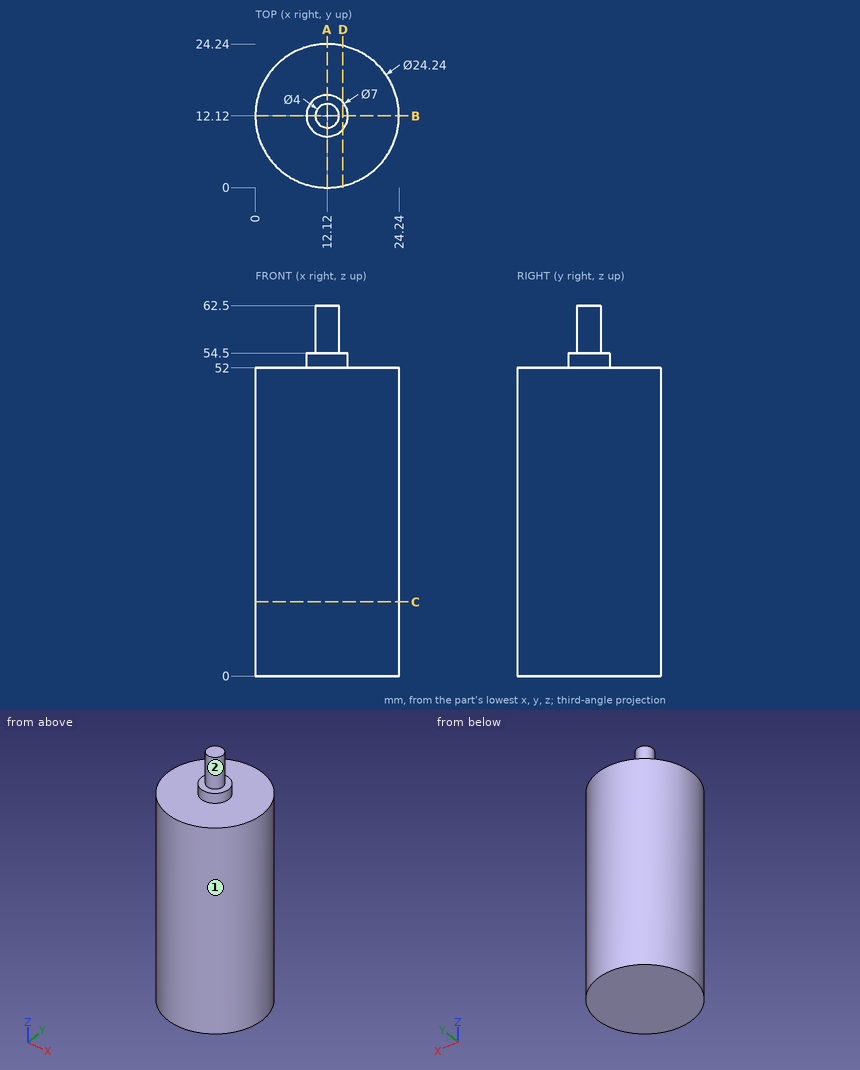
The figure shows three views and two pictorial views of one solid part (mm, origin at its lowest corner). Answer the questions. A direction names the side the tool comes from. Give positions to 0.01 mm unless a question says otherwise; leave off trailing zeros. Loops run counter-clockwise (first coordinate to the right, second up) from the corner with the lowest first, then second, coordinate; pieces in that order, holes last. Notation, with made-up numbers: (55.5, 42) -> (98.5, 42) arc R15 cw to (98.5, 61) -> close; hole circle Ø6 at (-23, 26.25). An arc over 180 degrees is marked (long way). Put each result on its own line as item: value. Start each with the question number.
Item 1: Which of the six approach directions +Z, -Z, +X, -X, +Y, -Y give full straight-line access (tool end or side, diameter ignored) to the marked faces 1 and 2?
Item 2: The part is cut by section A-A (x = 12.12). Give the vertices of the cut face in (y, z).
Item 3: Find the intervals of material crossed by L1, parallel to Z at x = 9.5, y = 11; L2, parallel to X at y = 12.5, z = 13.5; L3, parallel to Z at x = 5.75, y = 20.5, in increasing order. Write a range as [from, to].
Item 4: The part is cut by section C-C (z = 12.5). Give the vertices of the cut face in (x, y).
Item 5: Each of these flat-tipped pins is pushed along its axis until it touches: P1, Ø8, axis at x = 17.5, z = 49.5, coming from the +Y side; P2, Ø1.5, axis at y = 18, z = 9.5, coming from the +X side. Where does it stop, or does it pass through?
Item 6: The part is cut by section D-D (x = 14.75). Give the vertices of the cut face in (y, z), then the cut area to 3 significant figures.
Answers below:
1. face 1: +Z, -Z
1. face 2: +Z
2. outline: (0, 0) -> (24.24, 0) -> (24.24, 52) -> (15.62, 52) -> (15.62, 54.5) -> (14.12, 54.5) -> (14.12, 62.5) -> (10.12, 62.5) -> (10.12, 54.5) -> (8.62, 54.5) -> (8.62, 52) -> (0, 52) -> close
3. L1: [0, 54.5]
3. L2: [0.01, 24.23]
3. L3: [0, 52]
4. outline: circle Ø24.24 at (12.12, 12.12)
5. P1: y = 24.16
5. P2: x = 23.1
6. outline: (0.29, 0) -> (23.95, 0) -> (23.95, 52) -> (14.43, 52) -> (14.43, 54.5) -> (9.81, 54.5) -> (9.81, 52) -> (0.29, 52) -> close
6. area: 1,240 mm2
